```python
from build123d import *

# Parameters (mm, degrees)
F0_W     = 165.1
F0_H     = 76.2
F0_W_2   = 128.27
F0_H_2   = 26.67
F1_DEPTH = 9.525
F3_D     = 4.826
F4_R     = 1.5875
F5_R     = 6.35


with BuildPart() as f1:
    # F0 (on Front) → F1 (new body)
    with BuildSketch(Plane.XZ):
        Rectangle(F0_W, F0_H)
        Rectangle(F0_W_2, F0_H_2, mode=Mode.SUBTRACT)
    extrude(amount=F1_DEPTH)

    # F3 (through all)
    with Locations(Plane.XZ.offset(9.525)):
        with Locations((-69.85, 25.4), (69.85, 25.4), (69.85, -25.4), (-69.85, -25.4)):
            Hole(F3_D / 2)

    # F4
    f4_edges = [f1.edges().sort_by_distance(p)[0] for p in [
        (-64.135, -4.7625, 13.335),
        (-64.135, -4.7625, -13.335),
        (64.135, -4.7625, -13.335),
        (64.135, -4.7625, 13.335),
    ]]
    fillet(f4_edges, radius=F4_R)

    # F5
    f5_edges = [f1.edges().sort_by_distance(p)[0] for p in [
        (82.55, -4.7625, 38.1),
        (-82.55, -4.7625, 38.1),
        (82.55, -4.7625, -38.1),
        (-82.55, -4.7625, -38.1),
    ]]
    fillet(f5_edges, radius=F5_R)


solid = f1.part
```
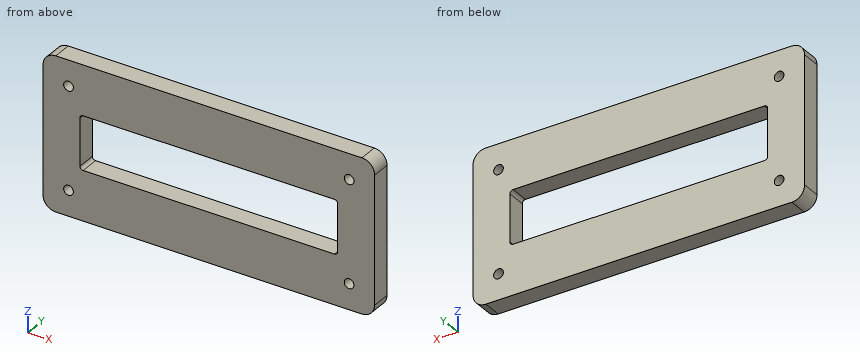
Read the model definition and answer for the solid it produces. Units are mm, in the model's axes. Give positions to 0.01 mm unless a question says otherwise; leave off trailing zeros. Write each loop counter-clockwise with the first axis right and the second up, starting at its lowest first coordinate (ties: lowest second). Pieces come first, ordered by that corner, then holes. Notation, with made-up numbers: (58, 69) -> (113, 69) arc R20 cw to (113, 93) -> close; hole circle Ø5 at (7.25, 8.5). An arc over 180 degrees is marked (long way). Answer in a Markdown table with one row per item.
1) Section B-B on x = 69.85 is taken. Give the vertices of the cut face in (y, z) (3 decimals), plus the area to 3 significant figures.
Results list:
| item | result |
|---|---|
| outline | (-9.525, -38.1) -> (0, -38.1) -> (0, -27.813) -> (-9.525, -27.813) -> close; (-9.525, -22.987) -> (0, -22.987) -> (0, 22.987) -> (-9.525, 22.987) -> close; (-9.525, 27.813) -> (0, 27.813) -> (0, 38.1) -> (-9.525, 38.1) -> close |
| area | 634 mm^2 |
2) Section C-C on y = -3.75 is taken. Count the separate pieces of the cut face and the enclosed holes in it, plus the area to 3 significant figures.
Results list:
| item | result |
|---|---|
| separate pieces | 1 |
| enclosed holes | 5 |
| area | 9,050 mm^2 |
3) Straight lines are drawn through the part: line 1 (Z direction, x = -69.85, y = -5.5); line 2 (X direction, y = -7.5, z = 2) (3 decimals); line 3 (Z direction, x = -14, y = -4.25) (3 decimals). For each, find the intervals that lie inside material, in ascending order. Write a range as [from, to].
Results list:
| item | result |
|---|---|
| line 1 | [-38.1, -27.81], [-22.99, 22.99], [27.81, 38.1] |
| line 2 | [-82.55, -64.135], [64.135, 82.55] |
| line 3 | [-38.1, -13.335], [13.335, 38.1] |
4) Section D-D on x = -40 is taken. Give the vertices of the cut face in (y, z) (3 decimals), plus the area to 3 significant figures.
Results list:
| item | result |
|---|---|
| outline | (-9.525, -38.1) -> (0, -38.1) -> (0, -13.335) -> (-9.525, -13.335) -> close; (-9.525, 13.335) -> (0, 13.335) -> (0, 38.1) -> (-9.525, 38.1) -> close |
| area | 472 mm^2 |
5) This flat-tipped pin is pushed along its axis until it touches: pin 1 Ø4.5 at (x, z) = (-69.85, 25.4) entering from -Y. Where does it stop, or does it pass through?
Results list:
| item | result |
|---|---|
| pin 1 | through |
6) Section A-A on z = 25.4 is taken. Give the vertices of the cut face in (x, y) (3 decimals).
Results list:
| item | result |
|---|---|
| outline | (-82.55, -9.525) -> (-72.263, -9.525) -> (-72.263, 0) -> (-82.55, 0) -> close; (-67.437, -9.525) -> (67.437, -9.525) -> (67.437, 0) -> (-67.437, 0) -> close; (72.263, -9.525) -> (82.55, -9.525) -> (82.55, 0) -> (72.263, 0) -> close |
